```python
from build123d import *

# Parameters (mm, degrees)
SKETCH1_W                = 14.2
SKETCH1_H                = 2.7
BOSS_EXTRUDE1_DEPTH      = 25
BOSS_EXTRUDE1_2_DEPTH    = 25
SKETCH2_W                = 17
SKETCH2_H                = 17
BOSS_EXTRUDE2_DEPTH      = 47.5
BOSS_EXTRUDE4_DEPTH      = 6
SKETCH6_W                = 42
SKETCH6_H                = 44
SKETCH6_W_2              = 38.5
SKETCH6_H_2              = 40.5
BOSS_EXTRUDE5_DEPTH      = 2
BOSS_EXTRUDE5_DEPTH_BACK = 6
SKETCH7_W                = 38.5
SKETCH7_H                = 40.5
SKETCH7_W_2              = 32.5
SKETCH7_H_2              = 34.5
BOSS_EXTRUDE6_DEPTH      = 2
BOSS_EXTRUDE7_DEPTH      = 3.25


with BuildPart() as part:
    # Sketch1 → Boss-Extrude1 (new body)
    with BuildSketch(Plane(origin=(0, 0, 0), x_dir=(1, 0, 0), z_dir=(0, 1, 0))):
        with Locations((0, -5.75)):
            Rectangle(SKETCH1_W, SKETCH1_H)
    extrude(amount=BOSS_EXTRUDE1_DEPTH)



with BuildPart() as body_2:
    # Sketch1 → Boss-Extrude1 2 (new body)
    with BuildSketch(Plane(origin=(0, 0, 0), x_dir=(1, 0, 0), z_dir=(0, 1, 0))):
        with Locations((0, 5.75)):
            Rectangle(SKETCH1_W, SKETCH1_H)
    extrude(amount=BOSS_EXTRUDE1_2_DEPTH)


with BuildPart() as part_1:
    add(part.part)

    add(body_2.part)  # Boss-Extrude2 merges body 2
    # Sketch2 → Boss-Extrude2 (add)
    with BuildSketch(Plane(origin=(0, 25, 0), x_dir=(1, 0, 0), z_dir=(0, 1, 0))):
        Rectangle(SKETCH2_W, SKETCH2_H)
    extrude(amount=BOSS_EXTRUDE2_DEPTH)

    # Sketch5 → Boss-Extrude4 (add, symmetric)
    with BuildSketch(Plane.XY):
        Polygon((-8.5, 72.5), (-5.035898385, 78.5), (18.5, 78.5), (18.5, 72.5), align=None)
    extrude(amount=BOSS_EXTRUDE4_DEPTH, both=True)

    # Sketch6 → Boss-Extrude5 (add, two sides)
    with BuildSketch(Plane(origin=(0, 78.5, 0), x_dir=(1, 0, 0), z_dir=(0, 1, 0))) as boss_extrude5_sk:
        with Locations((39.5, 0)):
            Rectangle(SKETCH6_W, SKETCH6_H)
        with Locations((39.5, 0)):
            Rectangle(SKETCH6_W_2, SKETCH6_H_2, mode=Mode.SUBTRACT)
    extrude(amount=BOSS_EXTRUDE5_DEPTH)
    extrude(boss_extrude5_sk.sketch, amount=-BOSS_EXTRUDE5_DEPTH_BACK)

    # Sketch7 → Boss-Extrude6 (add)
    with BuildSketch(Plane.XZ.offset(-72.5)):
        with Locations((39.5, 0)):
            Rectangle(SKETCH7_W, SKETCH7_H)
        with Locations((39.5, 0)):
            Rectangle(SKETCH7_W_2, SKETCH7_H_2, mode=Mode.SUBTRACT)
    extrude(amount=-BOSS_EXTRUDE6_DEPTH)

    # Sketch8 → Boss-Extrude7 (add, symmetric)
    with BuildSketch(Plane.XY):
        Polygon((16, 72.5), (8.5, 59.509618943), (8.5, 72.5), align=None)
    extrude(amount=BOSS_EXTRUDE7_DEPTH, both=True)


solid = part_1.part
```
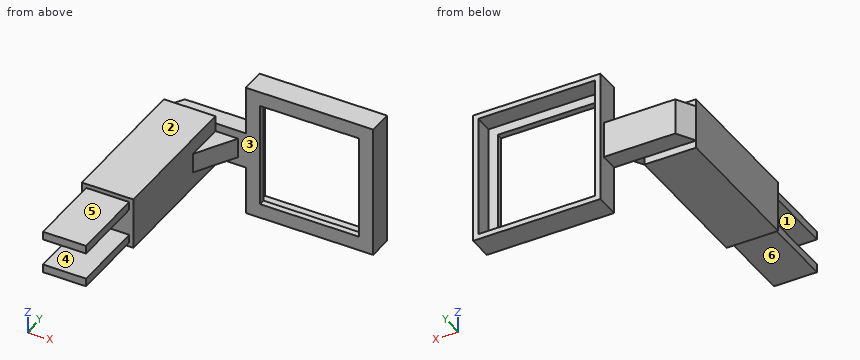
Can you work these out from the model? Positions are in its coordinate system, mm. Face numbers are marked on the shaded views. A direction names the side the tool comes from. Give positions to 0.01 mm unless a question says otherwise; leave off trailing zeros. Loops run counter-clockwise (first coordinate to the right, second up) from the corner with the lowest first, then second, coordinate; pieces in that order, holes last. Notation, with made-up numbers: M -18,-17.5 L -3,-17.5 A8 ccw -3,-6.5 Z; hole C -13,60 d2. An arc over 180 degrees is marked long. Answer in a Markdown table with one row per item.
1. If I drill on line 1 along Z through (x, y) = (1, 19.5); line 2 along Z through (x, y) = (36, 77); line 3 along Z through (x, y) = (-4, 48), over which ranges is the centre line in solid material (lowest first)?
Taken from the geometry:
| item | result |
|---|---|
| line 1 | z = -7.1 to -4.4, 4.4 to 7.1 |
| line 2 | z = -22 to -20.25, 20.25 to 22 |
| line 3 | z = -8.5 to 8.5 |
2. For pin 1 Ø6.5 at (x, y) = (1.5, 74) entering from -Z; pin 2 Ø1.2 at (x, z) = (-0.5, -7) entering from +Y; pin 3 Ø19 at (x, z) = (34.5, 10) entering from +Y; pin 4 Ø1 at (x, z) = (48, 16.5) entering from -Y, each with a flat end and sliding along its axis, tell me the tip position at first contact or that it passes through.
Taken from the geometry:
| item | result |
|---|---|
| pin 1 | stops at z = -8.5 |
| pin 2 | stops at y = 72.5 |
| pin 3 | stops at y = 74.5 |
| pin 4 | passes through |
3. Suppose I cut it at D-D on z = 14.5. Write out the boundary of the cut face in (x, y).
Taken from the geometry:
| item | result |
|---|---|
| outline | M 18.5,72.5 L 23.25,72.5 L 23.25,74.5 L 20.25,74.5 L 20.25,80.5 L 18.5,80.5 Z; M 55.75,72.5 L 60.5,72.5 L 60.5,80.5 L 58.75,80.5 L 58.75,74.5 L 55.75,74.5 Z |
4. Suppose I cut it at A-A on z = 2. Write out the boundary of the cut face in (x, y).
Taken from the geometry:
| item | result |
|---|---|
| outline | M -8.5,25 L 8.5,25 L 8.5,59.51 L 16,72.5 L 23.25,72.5 L 23.25,74.5 L 20.25,74.5 L 20.25,80.5 L 18.5,80.5 L 18.5,78.5 L -5.04,78.5 L -8.5,72.5 Z; M 55.75,72.5 L 60.5,72.5 L 60.5,80.5 L 58.75,80.5 L 58.75,74.5 L 55.75,74.5 Z |
5. Thinking about a two-plate mould opening in Z: for the marked faces 1, 2 and 3, which applies, released by +Z, released by -Z, zero draft, split by the parting line, or undercut?
Taken from the geometry:
| item | result |
|---|---|
| face 1 | undercut |
| face 2 | released by +Z |
| face 3 | zero draft |
6. Which directions (+Z, -Z, +X, -X, +Y, -Y) give clear straight access to the entire face, cutting with the end or side of a thin tool? Please do the marked faces 4, 5 and 6.
Taken from the geometry:
| item | result |
|---|---|
| face 4 | +X, -X, -Y |
| face 5 | +Z, +X, -X, -Y |
| face 6 | -Z, +X, -X, -Y |
7. Suppose I cut it at B-B on y = 9.5. Write out the boundary of the cut face in (x, z), plus the area to 3 significant figures.
Taken from the geometry:
| item | result |
|---|---|
| outline | M -7.1,-7.1 L 7.1,-7.1 L 7.1,-4.4 L -7.1,-4.4 Z; M -7.1,4.4 L 7.1,4.4 L 7.1,7.1 L -7.1,7.1 Z |
| area | 76.7 mm² |
8. Suppose I cut it at C-C on x = 44. Write out the boundary of the cut face in (y, z).
Taken from the geometry:
| item | result |
|---|---|
| outline | M 72.5,-22 L 80.5,-22 L 80.5,-20.25 L 74.5,-20.25 L 74.5,-17.25 L 72.5,-17.25 Z; M 72.5,17.25 L 74.5,17.25 L 74.5,20.25 L 80.5,20.25 L 80.5,22 L 72.5,22 Z |
